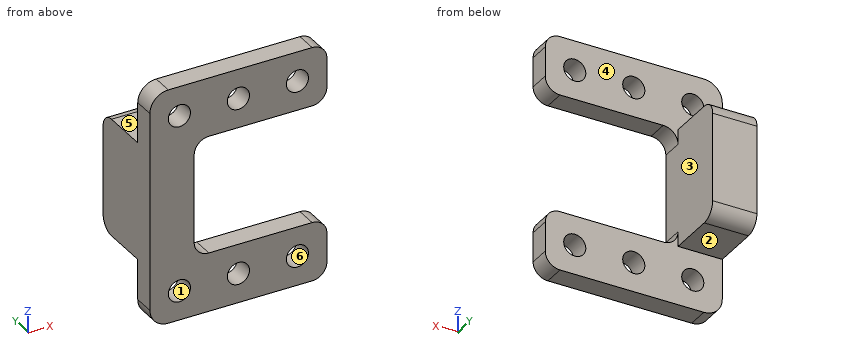
Autodesk Inventor part; units mm, degrees
ref_plane "YZ Plane" through (0, 0, 0) normal (1, 0, 0) x (0, 1, 0)
ref_plane "XZ Plane" through (0, 0, 0) normal (0, 1, 0) x (-1, 0, 0)
ref_plane "XY Plane" through (0, 0, 0) normal (0, 0, 1) x (1, 0, 0)
sketch "Sketch1" plane through (0, 0, 0) normal (1, 0, 0) x (0, 1, 0)
  line L0 (0, 0) -> (9.144, 0)
  line L1 (9.144, 0) -> (9.144, -25.4)
  line L2 (9.144, -25.4) -> (0, -25.4)
  line L3 (0, -25.4) -> (0, 0)
  dimension "d0" = 25.4
  dimension "d1" = 9.144
extrude "Extrusion1" add sketch "Sketch1" along normal blind 63.5
sketch "Sketch2" plane through (0, 9.144, 0) normal (0, 1, 0) x (1, 0, 0)
  line L0 (0, 25.4) -> (0, 0)
  line L1 (0, 12.7) -> (6.35, 12.7)
  line L2 (6.35, 12.7) -> (31.75, 12.7)
  line L3 (31.75, 12.7) -> (57.15, 12.7)
  circle A0 centre (6.35, 12.7) radius 4.7625
  circle A1 centre (31.75, 12.7) radius 4.7625
  circle A2 centre (57.15, 12.7) radius 4.7625
  dimension "d4" = 6.35
  dimension "d5" = 25.4
  dimension "d6" = 25.4
  dimension "d7" = 9.525
  dimension "d8" = 9.525
  dimension "d9" = 9.525
sketch "Sketch3" plane through (0, 0, 0) normal (-1, 0, 0) x (0, 0, 1)
  line L0 (-25.4, 0) -> (-25.4, 9.144)
  line L1 (0, 0) -> (-25.4, 0)
  line L2 (-25.4, 0) -> (-25.4, 9.144)
  line L3 (-25.4, 9.144) -> (0, 9.144)
  line L4 (0, 9.144) -> (0, 0)
extrude "Extrusion2" add sketch "Sketch3" along normal blind 3.175
extrude "Extrusion3" cut sketch "Sketch2" against normal blind 25.4
sketch "Sketch4" plane through (63.5, 0, 0) normal (1, 0, 0) x (0, 0, -1)
  line L0 (25.4, 0) -> (25.4, 9.144)
  line L1 (25.4, 9.144) -> (0, 9.144)
  line L2 (0, 9.144) -> (0, 0)
  line L3 (0, 0) -> (25.4, 0)
extrude "Extrusion4" add sketch "Sketch4" along normal blind 5.08
sketch "Sketch5" plane through (68.58, 0, 0) normal (1, 0, 0) x (0, 0, -1)
  line L0 (25.4, 9.144) -> (0, 9.144)
  line L1 (0, 9.144) -> (0, 0)
  line L2 (0, 0) -> (25.4, 0)
  line L3 (25.4, 0) -> (25.4, 9.144)
extrude "Extrusion5" add sketch "Sketch5" along normal blind 1.27
sketch "Sketch8" plane through (-3.175, 0, -25.4) normal (0, 0, -1) x (-1, 0, 0)
  line L0 (-73.025, 0) -> (0, 0)
  line L1 (0, 9.144) -> (-73.025, 9.144)
  line L2 (0, 0) -> (-15.875, 0)
  line L3 (-15.875, 0) -> (-15.875, 9.144)
  line L4 (-15.875, 9.144) -> (0, 9.144)
  line L5 (0, 9.144) -> (0, 0)
  line L6 (0, 9.144) -> (0, 0)
  point P0 (-3.175, 0)
  point P1 (0, 4.572)
  dimension "d24" = 15.875
extrude "Extrusion8" add sketch "Sketch8" along normal blind 50.8
sketch "Sketch9" plane through (-3.175, 0, 0) normal (-1, 0, 0) x (0, 0, 1)
  line L0 (0, 0) -> (0, 9.144)
  line L1 (0, 9.144) -> (-76.2, 9.144)
  line L2 (-76.2, 0) -> (-76.2, 9.144)
  line L3 (0, 0) -> (-76.2, 0)
extrude "Extrusion9" add sketch "Sketch9" along normal blind 3.175
sketch "Sketch10" plane through (69.85, 9.144, 0) normal (0, 1, 0) x (1, 0, 0)
  line L0 (-57.15, 25.4) -> (-57.15, 76.2)
  line L1 (-57.15, 76.2) -> (-66.675, 76.2)
  line L2 (-57.15, 76.2) -> (-76.2, 76.2)
  line L3 (-71.4375, 41.2761) -> (-61.9125, 41.2761)
  line L4 (-71.4375, 60.3261) -> (-61.9125, 60.3261)
  circle A0 centre (-66.675, 41.2761) radius 4.7625
  circle A1 centre (-66.675, 60.3261) radius 4.7625
  line L5 (-71.4375, 41.2761) -> (-71.4375, 60.3261)
  line L6 (-61.9125, 60.3261) -> (-61.9125, 41.2761)
  point P0 (-69.85, 0)
  dimension "d55" = 9.525
  dimension "d29" = 9.525
  dimension "d56" = 9.525
extrude "Extrusion10" add sketch "Sketch10" along normal blind 35.179
sketch "Sketch11" plane through (-3.175, 0, -76.2) normal (0, 0, -1) x (-1, 0, 0)
  line L0 (-15.875, 9.144) -> (3.175, 9.144)
  line L1 (-15.875, 9.144) -> (-15.875, 0)
  line L2 (-15.875, 0) -> (3.175, 0)
  line L3 (3.175, 9.144) -> (3.175, 0)
  point P0 (-3.175, 0)
extrude "Extrusion11" add sketch "Sketch11" along normal blind 25.4
sketch "Sketch13" plane through (12.7, 0, -25.4) normal (1, 0, 0) x (0, 0, -1)
  line L0 (0, 9.144) -> (76.2, 9.144)
  line L1 (-25.4, 0) -> (76.2, 0)
  line L2 (76.2, 9.144) -> (50.8, 9.144)
  line L3 (50.8, 9.144) -> (50.8, 0)
  line L4 (50.8, 0) -> (76.2, 0)
  line L5 (76.2, 0) -> (76.2, 9.144)
  dimension "d38" = 25.4
extrude "Extrusion12" add sketch "Sketch13" along normal blind 57.15
sketch "Sketch14" plane through (69.85, 9.144, 0) normal (0, 1, 0) x (1, 0, 0)
  circle A0 centre (-12.7, 12.7) radius 4.7625
  line L0 (-12.7, 12.7) -> (-12.7, 88.9)
  circle A1 centre (-38.1, 12.7) radius 4.7625
  line L1 (-38.1, 12.7) -> (-38.1, 88.9)
  circle A2 centre (-12.7, 88.9) radius 4.7625
  circle A3 centre (-38.1, 88.9) radius 4.7625
  circle A4 centre (-63.5, 12.7) radius 4.7625
  line L2 (-63.5, 12.7) -> (-63.5, 88.9)
  circle A5 centre (-63.5, 88.9) radius 4.7625
  point P0 (-69.85, 0)
  dimension "d42" = 76.2
  dimension "d43" = 76.2
  dimension "d44" = 9.525
  dimension "d45" = 9.525
  dimension "d46" = 9.525
extrude "Extrusion13" cut sketch "Sketch14" against normal blind 20.6375 contours A2 | A3 | A5
fillet "Fillet2" radius 7.9375 2 edges at (-6.35, 4.572, -101.6) (-6.35, 4.572, 0)
sketch "Sketch15" plane through (69.85, 9.144, 0) normal (0, 1, 0) x (1, 0, 0)
  line L0 (0, 25.4) -> (-57.15, 25.4)
  line L1 (-57.15, 25.4) -> (-76.2, 25.4)
  line L2 (-76.2, 7.9375) -> (-76.2, 93.6625)
  line L3 (-57.15, 25.4) -> (-57.15, 76.2)
  line L4 (-57.15, 76.2) -> (-76.2, 76.2)
  line L5 (-71.4375, 31.7511) -> (-71.4375, 69.8511)
  line L6 (-61.9125, 69.8511) -> (-61.9125, 31.7511)
  arc A0 (-71.4375, 31.7511) -> (-61.9125, 31.7511) centre (-66.675, 31.7511) ccw
  arc A1 (-61.9125, 69.8511) -> (-71.4375, 69.8511) centre (-66.675, 69.8511) ccw
  arc A2 (-71.4375, 41.2761) -> (-61.9125, 41.2761) centre (-66.675, 41.2761) ccw
  arc A3 (-61.9125, 60.3261) -> (-71.4375, 60.3261) centre (-66.675, 60.3261) ccw
  point P0 (-69.85, 0)
extrude "Extrusion14" add sketch "Sketch15" along normal blind 26.035 contours L1 L2 L4 L3 | L5 A2 L6 A0 | L5 A1 L6 A3
fillet "Fillet3" radius 6.35 2 edges at (3.175, 35.179, -76.2) (3.175, 35.179, -25.4)
sketch "Sketch16" plane through (-1.5875, 44.323, -60.3261) normal (-1, 0, 0) x (0, 0, 1)
  arc A0 (-9.5239, -9.144) -> (-15.8739, -15.494) centre (-9.5239, -15.494) ccw
  line L0 (-9.5239, -9.144) -> (49.3517, -9.144)
  line L1 (49.3517, -9.144) -> (49.3517, 6.1013)
  line L2 (49.3517, 6.1013) -> (-9.5239, 6.1013)
  line L3 (-9.5239, 6.1013) -> (-9.5239, -9.144)
  point P0 (60.3261, -44.323)
extrude "Extrusion15" cut sketch "Sketch16" against normal blind 21.971
fillet "Fillet5" radius 6.35 6 edges at (12.7, 4.572, -76.2) (12.7, 4.572, -25.4) (69.85, 4.572, -76.2) (69.85, 4.572, -101.6) (69.85, 4.572, -25.4) (69.85, 4.572, 0)
properties part number "CH-1-03-RearGearboxSpacer_01"
For this review, take the finished solid that the model builds, in its own axes (mm). Face numbers are marked on the shaded views. A direction names the side the tool comes from. Round coordinates to 2 decimals unless told otherwise and drop trailing zeros. Write each loop counter-clockwise with the first axis right and the second up, starting at its lowest first coordinate (ties: lowest second). Pieces come first, ordered by that corner, then holes. Notation, with made-up numbers: M 20.5,58.5 L 42.5,58.5 A5 ccw 42.5,62.5 Z; hole C -18,26 d5. An arc over 180 degrees is marked long. Write item = value, one per line. Start each with the question number.
(1) We need section D-D (x = 7.5). Give the boundary of the cut face in (y, z).
(2) For the marked faces 1, 2 and 3, list the 3-axis set-ups (+Z, -Z, +X, -X, +Y, -Y) from which the entire face can be reached by the end or side of a thin tool; tool diameter is ignored.
(3) The part is to be moulded in two halves that separate along Z. For the marked faces 4, 5 and 6, say which applies: +Z half, -Z half, draft (parallel to the pull), parting line (faces both ways), or undercut.
(4) We need section C-C (x = 31.75). Give the boundary of the cut face in (y, z), then the cut area to 3 significant figures.
(5) Clearance check with flat-ended pins moving along their axes: pin 1 Ø7.5 at (x, y) = (44, 6) entering from +Z; pin 2 Ø7.5 at (x, z) = (6.35, -88.9) entering from +Y; pin 3 Ø11 at (x, z) = (57.15, -12.7) entering from +Y; pin 4 Ø9.5 at (x, y) = (6.5, 16) entering from +Z. State where each tip first meets the part, or that it passes through.
(6) We need section B-B (z = -88.9). Give the boundary of the cut face in (x, y), then the cut area to 3 significant figures.
(7) For line 1 along X through (y, z) = (4.5, -88.9); line 2 along Z through (x, y) = (31.75, 7.25); line 3 along Z through (x, y) = (6, 3), list the stretches that pass through material, from the lowest coordinate up.
(8) We need section A-A (x = 49). Give the boundary of the cut face in (y, z), then the cut area to 3 significant figures.
Results found:
q1.outline = M 0,-101.6 L 9.14,-101.6 L 9.14,-93.52 L 0,-93.52 Z; M 0,-84.28 L 9.14,-84.28 L 9.14,-76.2 L 28.83,-76.2 A6.35 ccw 35.18,-69.85 L 35.18,-31.75 A6.35 ccw 28.83,-25.4 L 9.14,-25.4 L 9.14,-17.32 L 0,-17.32 Z; M 0,-8.08 L 9.14,-8.08 L 9.14,0 L 0,0 Z
q2.face_1 = +Y, -Y
q2.face_2 = -Z, +X, -X, +Y
q2.face_3 = +X, +Y
q3.face_4 = draft
q3.face_5 = +Z half
q3.face_6 = undercut
q4.outline = M 0,-101.6 L 9.14,-101.6 L 9.14,-93.66 L 0,-93.66 Z; M 0,-84.14 L 9.14,-84.14 L 9.14,-76.2 L 0,-76.2 Z; M 0,-25.4 L 9.14,-25.4 L 9.14,-17.46 L 0,-17.46 Z; M 0,-7.94 L 9.14,-7.94 L 9.14,0 L 0,0 Z
q4.area = 290 mm²
q5.pin_1 = 0
q5.pin_2 = through
q5.pin_3 = 9.14
q5.pin_4 = -25.4
q6.outline = M -6.35,0 L 1.59,0 L 1.59,9.14 L -6.35,9.14 Z; M 11.11,0 L 26.99,0 L 26.99,9.14 L 11.11,9.14 Z; M 36.51,0 L 52.39,0 L 52.39,9.14 L 36.51,9.14 Z; M 61.91,0 L 69.85,0 L 69.85,9.14 L 61.91,9.14 Z
q6.area = 435 mm²
q7.line_1 = -6.35 to 1.59, 11.11 to 26.99, 36.51 to 52.39, 61.91 to 69.85
q7.line_2 = -101.6 to -93.66, -84.14 to -76.2, -25.4 to -17.46, -7.94 to 0
q7.line_3 = -101.6 to -93.65, -84.15 to -17.45, -7.95 to 0
q8.outline = M 0,-101.6 L 9.14,-101.6 L 9.14,-76.2 L 0,-76.2 Z; M 0,-25.4 L 9.14,-25.4 L 9.14,0 L 0,0 Z
q8.area = 465 mm²
